Autodesk Inventor part; units mm, degrees
ref_plane "YZ Plane" through (0, 0, 0) normal (1, 0, 0) x (0, 1, 0)
ref_plane "XZ Plane" through (0, 0, 0) normal (0, 1, 0) x (-1, 0, 0)
ref_plane "XY Plane" through (0, 0, 0) normal (0, 0, 1) x (1, 0, 0)
sketch "スケッチ1" plane through (0, 0, 0) normal (0, 1, 0) x (-1, 0, 0)
  line L0 (0, 0) -> (-300, 0)
  line L1 (-300, 0) -> (-300, -35)
  line L2 (-300, -35) -> (0, -35)
  line L3 (0, -35) -> (0, 0)
  arc A0 (-17.5, -35) -> (-17.5, 0) centre (-17.5, -17.5) ccw
  point P0 (-17.5, -17.5)
  dimension "d0" = 300
  dimension "d1" = 35
  dimension "d2" = 17.5
  dimension "d3" = 17.5
  dimension "d43" = 17.5
extrude "押し出し1" add sketch "スケッチ1" along normal blind 3 contours A0 L2 L1 L0
sketch "スケッチ2" plane through (0, 3, 0) normal (0, 1, 0) x (1, 0, 0)
  arc A0 (17.5, 35) -> (17.5, 0) centre (17.5, 17.5) ccw
  line L0 (300, 35) -> (17.5, 35)
  point P0 (0, 0)
  point P1 (0, 17.5)
hole "穴1" at (17.5, 3, -17.5) direction (0, -1, 0) diameter 16 end through all
sketch "スケッチ3" plane through (0, 3, 0) normal (0, 1, 0) x (1, 0, 0)
  line L0 (300, 0) -> (300, 35)
  arc A0 (17.5, 35) -> (17.5, 0) centre (17.5, 17.5) ccw construction
  line L1 (17.5, 17.5) -> (300, 17.5) construction
  line L2 (300, 0) -> (300, 35) construction
  point P0 (0, 0)
  point P1 (57.5, 17.5)
  point P2 (67.5, 17.5)
  point P3 (77.5, 17.5)
  point P4 (87.5, 17.5)
  point P5 (97.5, 17.5)
  point P6 (107.5, 17.5)
  point P7 (117.5, 17.5)
  point P8 (127.5, 17.5)
  point P9 (137.5, 17.5)
  point P10 (147.5, 17.5)
  point P11 (157.5, 17.5)
  point P12 (167.5, 17.5)
  point P13 (177.5, 17.5)
  point P14 (187.5, 17.5)
  point P15 (197.5, 17.5)
  point P16 (207.5, 17.5)
  point P17 (217.5, 17.5)
  point P18 (227.5, 17.5)
  point P19 (237.5, 17.5)
  point P20 (247.5, 17.5)
  point P21 (257.5, 17.5)
  point P22 (267.5, 17.5)
  point P23 (277.5, 17.5)
  point P24 (287.5, 17.5)
  dimension "d108" = 40
  dimension "d111" = 10
hole "穴7" at (57.5, 3, -17.5) at (67.5, 3, -17.5) at (77.5, 3, -17.5) at (87.5, 3, -17.5) at (97.5, 3, -17.5) at (107.5, 3, -17.5) at (117.5, 3, -17.5) at (127.5, 3, -17.5) at (137.5, 3, -17.5) at (147.5, 3, -17.5) at (157.5, 3, -17.5) at (167.5, 3, -17.5) at (177.5, 3, -17.5) at (187.5, 3, -17.5) at (197.5, 3, -17.5) at (207.5, 3, -17.5) at (217.5, 3, -17.5) at (227.5, 3, -17.5) at (237.5, 3, -17.5) at (247.5, 3, -17.5) at (257.5, 3, -17.5) at (267.5, 3, -17.5) at (277.5, 3, -17.5) at (287.5, 3, -17.5) direction (0, -1, 0) diameter 3.2 end through all
sketch "スケッチ10" plane through (0, 3, 0) normal (0, 1, 0) x (1, 0, 0)
  circle A0 centre (17.5, 17.5) radius 8 construction
  circle A1 centre (17.5, 17.5) radius 12.5 construction
  point P0 (0, 0)
  point P1 (17.5, 5)
  point P2 (30, 17.5)
  point P3 (17.5, 30)
  point P4 (5, 17.5)
  dimension "d123" = 25
  dimension "d126" = 360
hole "穴8" at (17.5, 3, -5) at (30, 3, -17.5) at (17.5, 3, -30) at (5, 3, -17.5) direction (0, -1, 0) diameter 3.2 end through all
properties part number "shoulder1_bottom_plate" material "アルミニウム 5052"
For this review, take the finished solid that the model builds, in its own axes (mm). Round coordinates to 2 decimals unless told otherwise and drop trailing zeros. One line per question, with ' | ' between items. Start each with the question number.
(1) Add section A-A, the plane y = 0.65. Give the number of separate pieces and of enclosed holes in the cut face, plus the area to 3 significant figures.
(2) For line 1 along Z through (x, y) = (17.5, 0.7); line 2 along Z through (x, y) = (127.5, 1.05); line 3 along X through (y, z) = (1.2, -30.5), list the stretches that pass through material, from the lowest coordinate up. Write a range as from..to.
(3) Mouldability with a two-part tool opening along Z and no side actions: class faces 1 (the face through (0.004, 1.479, -17.115)), 2 (the face through (22.368, 1.479, -23.849)), 3 (the face through (152, 3, -17)) as released by +Z, released by -Z, zero draft, split by the parting line, or undercut.
(4) Insertion check: P1, Ø3.5, axis at x = 67.5, z = -17.5, coming from the -Y side. The pin has a flat end and moves straight along its axis. Give the tip position at first contact, or say it passes through.
Answer list:
1) separate pieces: 1 | enclosed holes: 29 | area: 9,940 mm²
2) line 1: -35..-31.6, -28.4..-25.5, -9.5..-6.6, -3.4..0 | line 2: -35..-19.1, -15.9..0 | line 3: 5.78..15.98, 19.02..300
3) face 1: split by the parting line | face 2: undercut | face 3: zero draft
4) P1: y = 0
